Can you work these out from the model? Positions are in its coordinate system, mm. A direction names the side the tool comes from. Coordinates: 2 decimals unless noted, no trailing zeros. Order: outer loops, then holes, each group sorted by start corner. A loop starts at its lowest first (then second) coordinate and runs counter-clockwise, first axis right, second up. Notation, with made-up numbers: M 84,50.5 L 122,50.5 A35 cw 122,87.5 Z; hole C -36.5,-16 d3. An arc over 180 degrees is marked long. Answer as a JSON object with one key per item and string values.
Autodesk Inventor part; units mm, degrees
ref_plane "Work Plane1" through (0, 0, -65) normal (0, 0, -1) x (-1, 0, 0)
ref_plane "YZ Plane" through (0, 0, 0) normal (1, 0, 0) x (0, 1, 0)
ref_plane "XZ Plane" through (0, 0, 0) normal (0, 1, 0) x (-1, 0, 0)
sketch "Sketch1" plane through (0, 0, 0) normal (0, 0, 1) x (1, 0, 0)
  line L0 (0, 37.5) -> (8.5, 37.5) construction
  circle A0 centre (8.5, 37.5) radius 2
  line L1 (8.5, 37.5) -> (-8.5, 37.5) construction
  line L2 (-8.5, 37.5) -> (-8.5, -37.5) construction
  line L3 (-8.5, -37.5) -> (8.5, -37.5) construction
  line L4 (8.5, -37.5) -> (8.5, 37.5) construction
  circle A1 centre (8.5, -37.5) radius 2
  line L5 (-8.5, 37.5) -> (8.5, -37.5) construction
  line L6 (-14.9, 32.5) -> (14.9, 32.5)
  line L7 (14.9, 32.5) -> (14.9, -32.5)
  line L8 (14.9, -32.5) -> (-14.9, -32.5)
  line L9 (-14.9, 32.5) -> (14.9, -32.5) construction
  line L10 (14.9, 32.5) -> (-14.9, -32.5) construction
  circle A2 centre (-8.5, -37.5) radius 2
  circle A3 centre (-8.5, 37.5) radius 2
  arc A4 (-8.5, -20) -> (-9.1777, -20.0184) centre (-8.5, -32.5) ccw
  line L11 (0, 19) -> (0, 0) construction
  line L12 (0, 32.5) -> (0, 19) construction
  line L13 (35, 25.75) -> (35, -74.25)
  line L14 (35, -74.25) -> (-35, -74.25)
  line L15 (-35, -74.25) -> (-35, -32.5)
  arc A5 (35, 25.75) -> (0, 60.75) centre (0, 25.75) ccw
  line L16 (0, 60.75) -> (-35, 60.75)
  line L17 (-35, 60.75) -> (-35, 32.5)
  line L18 (-14.9, -32.5) -> (-35, -32.5)
  line L19 (-14.9, 32.5) -> (-35, 32.5)
  point P0 (8.5, -32.5)
  dimension "d0" = 8.5
  dimension "d1" = 4
  dimension "d2" = 17
  dimension "d3" = 75
  dimension "d4" = 4
  dimension "d5" = 29.8
  dimension "d6" = 65
  dimension "d7" = 4
  dimension "d8" = 4
  dimension "d9" = 13.5
  dimension "d12" = 100
  dimension "d15" = 35
extrude "Extrusion1" add sketch "Sketch1" along normal blind 10
ref_plane "Work Plane1" through (0, 0, -65) normal (0, 0, -1) x (-1, 0, 0)
sketch "Sketch2" plane through (0, 0, -65) normal (0, 0, -1) x (-1, 0, 0)
  line L0 (35, -32.5) -> (35, -74.25)
  arc A0 (0, 60.75) -> (-35, 25.75) centre (0, 25.75) ccw
  line L1 (-35, -74.25) -> (-35, 25.75)
  line L2 (35, -74.25) -> (-35, -74.25)
  circle A1 centre (-8.5, -37.5) radius 2
  circle A2 centre (8.5, -37.5) radius 2
  circle A3 centre (8.5, 37.5) radius 2
  circle A4 centre (-8.5, 37.5) radius 2
  line L3 (-14.9, 32.5) -> (-14.9, -32.5)
  line L4 (35, 32.5) -> (-14.9, 32.5)
  line L5 (-14.9, -32.5) -> (35, -32.5)
  line L6 (35, 60.75) -> (35, 32.5)
  line L7 (0, 60.75) -> (35, 60.75)
  point P0 (0, 0)
extrude "Extrusion2" add sketch "Sketch2" along normal blind 10
sketch "Sketch3" plane through (0, 0, 0) normal (0, 0, -1) x (-1, 0, 0)
  line L0 (-35, -74.25) -> (-35, 25.75)
  line L1 (-35, -74.25) -> (-25, -74.25)
  line L2 (-25, -74.25) -> (-25, -4.25)
  line L3 (-25, -4.25) -> (-35, -4.25)
  line L4 (-35, -4.25) -> (-35, -74.25)
  line L5 (35, -74.25) -> (-35, -74.25)
  line L6 (-14.9, -32.5) -> (35, -32.5)
  line L7 (35, -74.25) -> (25, -74.25)
  line L8 (25, -74.25) -> (25, -32.5)
  line L9 (25, -32.5) -> (35, -32.5)
  line L10 (35, -32.5) -> (35, -74.25)
  line L11 (35, 60.75) -> (35, 32.5)
  line L12 (35, 32.5) -> (-14.9, 32.5)
  line L13 (35, 60.75) -> (25, 60.75)
  line L14 (25, 60.75) -> (25, 32.5)
  line L15 (25, 32.5) -> (35, 32.5)
  line L16 (35, 32.5) -> (35, 60.75)
  point P0 (0, 0)
  point P1 (-35, -4.25)
  dimension "d19" = 10
  dimension "d23" = 70
  dimension "d24" = 10
  dimension "d25" = 10
extrude "Extrusion3" add sketch "Sketch3" along normal up to next
sketch "Sketch4" plane through (35, 0, 10) normal (1, 0, 0) x (0, 0, -1)
  line L0 (85, 25.75) -> (85, -74.25)
  line L1 (0, -32.5) -> (0, -74.25)
  line L2 (85, -74.25) -> (0, -74.25)
  line L3 (0, -74.25) -> (0, -44.25)
  line L4 (0, -44.25) -> (85, -44.25)
  line L5 (85, -44.25) -> (85, -74.25)
  line L6 (0, -74.25) -> (85, -74.25) construction
  line L7 (85, -44.25) -> (0, -74.25) construction
  line L8 (42.5, -59.25) -> (57.5, -59.25) construction
  line L9 (42.5, -59.25) -> (27.5, -59.25) construction
  circle A0 centre (57.5, -59.25) radius 2.5
  circle A1 centre (27.5, -59.25) radius 2.5
  point P0 (10, 0)
  dimension "d26" = 30
  dimension "d27" = 15
  dimension "d28" = 15
  dimension "d29" = 5
  dimension "d30" = 5
extrude "Extrusion4" cut sketch "Sketch4" against normal blind 90 contours A0 | A1
properties part number "Joint_3_House" material "Acrylic, Clear"
Item 1: I'm going to push flat-ended pins straight in: pin 1 (5 mm diameter, centred on y = -14, z = 6.5, fed in from -X); pin 2 (6 mm diameter, centred on y = -59.25, z = -47.5, fed in from +X); pin 3 (14 mm diameter, centred on y = 42.5, z = -44, fed in from +X). Where does each tip first touch, or does it pass through?
Answers follow:
{"pin 1": "stops at x = 14.9", "pin 2": "stops at x = 35", "pin 3": "stops at x = -25"}
Item 2: Please list where these lines run through material, in increasing order: line 1 (Z direction, x = -31, y = -59); line 2 (Y direction, x = -8.5, z = 5); line 3 (Y direction, x = -28, z = -6.5).
Answers follow:
{"line 1": "z = -75 to -49.99, -45.01 to -19.99, -15.01 to 10", "line 2": "y = -74.25 to -39.5, -35.5 to -32.5, 32.5 to 35.5, 39.5 to 60.75", "line 3": "y = -74.25 to -32.5, 32.5 to 60.75"}
Item 3: If we mould it in two halves opening along Y, with no side actions, what happens to faces 6 (the cylindrical face through (25.019, 50.225, -69.93)), 7 (the flat face through (-25, -54, -32)), 8 (the flat face through (14.9, 0, -70))? For each: pulls with the +Y half, pulls with the -Y half, needs draft (parallel to the pull), parting line crosses it, or undercut.
Answers follow:
{"face 6": "pulls with the +Y half", "face 7": "needs draft", "face 8": "undercut"}
Item 4: I want a section at B-B, the plane x = -4. Write out the boundary of the cut face in (y, z).
Answers follow:
{"outline": "M -74.25,-75 L -32.5,-75 L -32.5,-65 L -74.25,-65 Z; M -74.25,0 L -32.5,0 L -32.5,10 L -74.25,10 Z; M 32.5,-75 L 60.75,-75 L 60.75,-65 L 32.5,-65 Z; M 32.5,0 L 60.75,0 L 60.75,10 L 32.5,10 Z"}
Item 5: I want a section at C-C, the plane z = -47.5. Write out the boundary of the cut face in (x, y), plus the area to 3 significant figures.
Answers follow:
{"outline": "M -35,-74.25 L -25,-74.25 L -25,-61.75 L -35,-61.75 Z; M -35,-56.75 L -25,-56.75 L -25,-32.5 L -35,-32.5 Z; M -35,32.5 L -25,32.5 L -25,60.75 L -35,60.75 Z; M 25,-74.25 L 35,-74.25 L 35,-61.75 L 25,-61.75 Z; M 25,-56.75 L 35,-56.75 L 35,-4.25 L 25,-4.25 Z", "area": "1,300 mm^2"}
Item 6: I want a section at D-D, the plane z = -22. Write out the boundary of the cut face in (x, y), plus the area to 3 significant figures.
Answers follow:
{"outline": "M -35,-74.25 L -25,-74.25 L -25,-32.5 L -35,-32.5 Z; M -35,32.5 L -25,32.5 L -25,60.75 L -35,60.75 Z; M 25,-74.25 L 35,-74.25 L 35,-4.25 L 25,-4.25 Z", "area": "1,400 mm^2"}
Item 7: I want a section at A-A, the plane y = -59.25. Write out the boundary of the cut face in (x, z).
Answers follow:
{"outline": "M -35,-75 L 35,-75 L 35,-50 L 25,-50 L 25,-65 L -25,-65 L -25,-50 L -35,-50 Z; M -35,-45 L -25,-45 L -25,-20 L -35,-20 Z; M -35,-15 L -25,-15 L -25,0 L 25,0 L 25,-15 L 35,-15 L 35,10 L -35,10 Z; M 25,-45 L 35,-45 L 35,-20 L 25,-20 Z"}
Item 8: Which directions (+Z, -Z, +X, -X, +Y, -Y) give clear straight access to the entire face, cutting with the end or side of a thin tool? Please do faces 1 (the flat face through (19, -6, -65)), 2 (the flat face through (-26, -32.5, -33)), 3 (the flat face through (-25, 47, -32)), 4 (the cylindrical face through (8.934, -35.548, -69.93)), 5 (the flat face through (30, -4.25, -32)).
Answers follow:
{"face 1": "+Y", "face 2": "+Z, -Z, -X", "face 3": "+X, +Y, -Y", "face 4": "+Z, -Z", "face 5": "+X, -X, +Y"}
